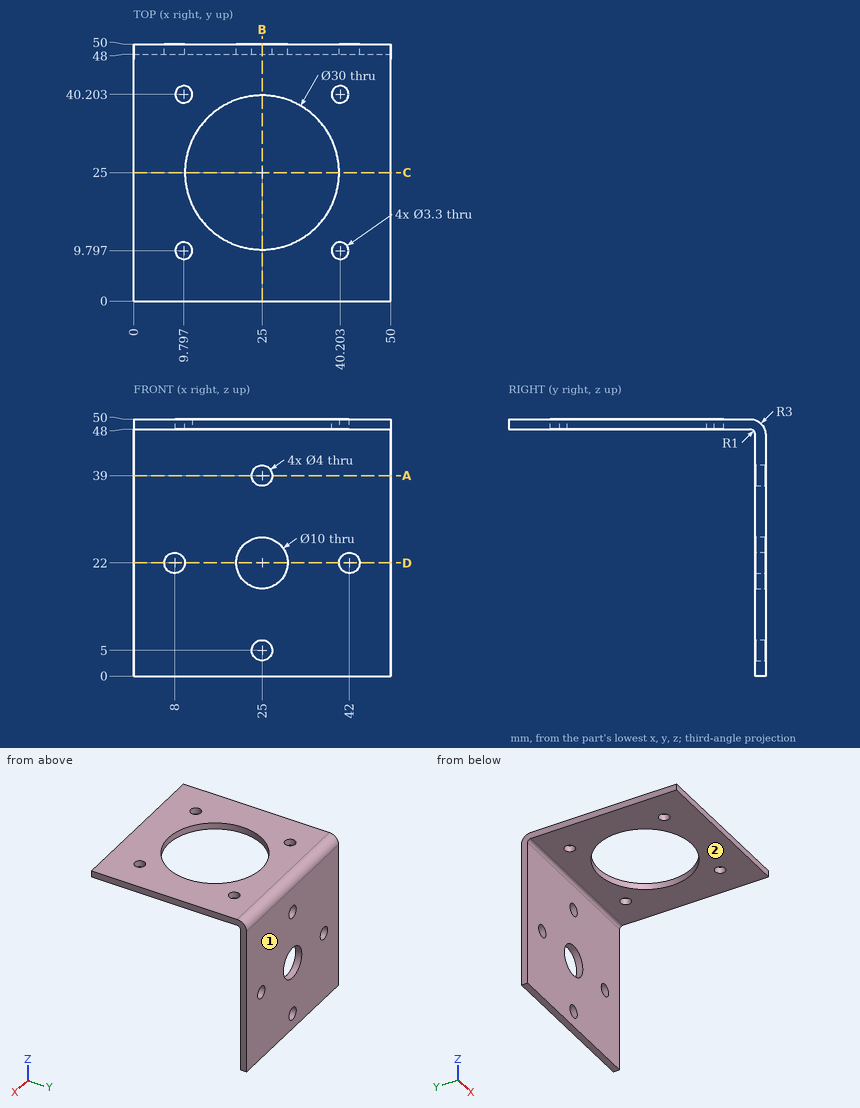
Print and shaded views of the part. All mm, measured from the part's lowest x, y and z. A direction names the side the tool comes from. Coordinates: 2 decimals unless noted, no trailing zeros. Order: outer loops, then holes, each group sorted by start corner. A loop starts at its lowest first (then second) coordinate and runs counter-clockwise, first axis right, second up. Notation, with made-up numbers: (47.5, 80) - (97.5, 80) arc R20 cw to (97.5, 99) - close; hole circle Ø4 at (6.5, 47.25). An arc over 180 degrees is marked (long way). Return JSON: item names as keys, results as strings. Group by question number.
Item 1: Cut at D-D (z = 22). List the corners of the cut face in (x, y).
Item 2: Cut at B-B (x = 25). List the corners of the cut face in (y, z).
Item 3: Which spindle directions (+Z, -Z, +X, -X, +Y, -Y) get a long thin tool onto all of the face, cutting with end or side? Do the marked faces 1 and 2. Say none if no direction does.
Item 4: Pin check, flat tips, straight feed: pin 1 (12 mm diameter, centred on x = 8.5, z = 38.5, fed in from -Y); pin 2 (1.5 mm diameter, centred on x = 43, y = 32, fed in from -Z). Stop position of each tip, or through.
Item 5: Cut at A-A (z = 39). List the corners of the cut face in (x, y), plus the area to 3 significant figures.
Item 6: Drill centre lines: probe 1 along X at (y, z) = (49.3, 5); probe 2 along Z at (x, y) = (44, 23). Where is each one in solid material? Low to high. Write a range as from..to.
Item 7: Cut at C-C (y = 25). List the corners of the cut face in (x, z), plus the area to 3 significant figures.
Check values:
{
 "1": {"outline": "(0, 48) - (6, 48) - (6, 50) - (0, 50) - close; (10, 48) - (20, 48) - (20, 50) - (10, 50) - close; (30, 48) - (40, 48) - (40, 50) - (30, 50) - close; (44, 48) - (50, 48) - (50, 50) - (44, 50) - close"},
 "2": {"outline": "(0, 48) - (10, 48) - (10, 50) - (0, 50) - close; (40, 48) - (47, 48) arc R1 cw to (48, 47) - (48, 41) - (50, 41) - (50, 47) arc R3 ccw to (47, 50) - (40, 50) - close; (48, 0) - (50, 0) - (50, 3) - (48, 3) - close; (48, 7) - (50, 7) - (50, 17) - (48, 17) - close; (48, 27) - (50, 27) - (50, 37) - (48, 37) - close"},
 "3": {"face 1": "+Z, -Z, +X, -X, +Y", "face 2": "-Z, +X, -X, -Y"},
 "4": {"pin 1": "stops at y = 48", "pin 2": "stops at z = 48"},
 "5": {"outline": "(0, 48) - (23, 48) - (23, 50) - (0, 50) - close; (27, 48) - (50, 48) - (50, 50) - (27, 50) - close", "area": "92.0 mm2"},
 "6": {"probe 1": "x = 0..23, 27..50", "probe 2": "z = 48..50"},
 "7": {"outline": "(0, 48) - (10, 48) - (10, 50) - (0, 50) - close; (40, 48) - (50, 48) - (50, 50) - (40, 50) - close", "area": "40.0 mm2"}
}
